Verification items for the finished model (mm, model axes). A direction names the side the tool comes from. Give positions to 0.01 mm unless a question says otherwise; leave off trailing zeros. Order: outer loops, then holes, each group sorted by start corner. A loop starts at its lowest first (then second) coordinate and runs counter-clockwise, first axis right, second up. Notation, with made-up numbers: (58, -28.75) - (96, -28.75) arc R14 ccw to (96, -4.75) - close; hole circle Ø6 at (11, 22.5). An arc over 180 degrees is marked (long way). Answer as a JSON object with one key per item and string values.
```python
from build123d import *

# Parameters (mm, degrees)
SALIENTE_EXTRUIR1_DEPTH = 60
CHAFL_N1_SIZE           = 1.5
CROQUIS3_R              = 2.25
CORTAR_EXTRUIR2_DEPTH   = 4.5


with BuildPart() as part:
    # Croquis1 → Saliente-Extruir1 (new body, symmetric)
    with BuildSketch(Plane(origin=(0, 0, 0), x_dir=(0, 0, -1), z_dir=(1, 0, 0))):
        Polygon((0, -23.75), (0, 23.75), (-21, 23.75), (-21, 20.25), (-3.5, 20.25), (-3.5, -20.25), (-21, -20.25), (-21, -23.75), align=None)
    extrude(amount=SALIENTE_EXTRUIR1_DEPTH, both=True)

    # Chaflán1
    chafl_n1_edges = [part.edges().sort_by_distance(p)[0] for p in [
        (0, 23.75, 0),
        (0, -23.75, 0),
    ]]
    chamfer(chafl_n1_edges, length=CHAFL_N1_SIZE)

    # Croquis3 → Cortar-Extruir2 (cut, through all)
    with BuildSketch(Plane.XY.offset(3.5)):
        with Locations((-40, 0.25)):
            Circle(CROQUIS3_R)
        with Locations((40, 0.25)):
            Circle(CROQUIS3_R)
    extrude(amount=-CORTAR_EXTRUIR2_DEPTH, mode=Mode.SUBTRACT)


solid = part.part
```
(1) Section check A-A (z = 10.5). Record the cut outline in (x, y), then the cut area to 3 significant figures.
Computed values:
{"outline": "(-60, -23.75) - (60, -23.75) - (60, -20.25) - (-60, -20.25) - close; (-60, 20.25) - (60, 20.25) - (60, 23.75) - (-60, 23.75) - close", "area": "840 mm²"}
(2) Section check D-D (x = 34). Record the cut outline in (y, z).
Computed values:
{"outline": "(-23.75, 1.5) - (-22.25, 0) - (22.25, 0) - (23.75, 1.5) - (23.75, 21) - (20.25, 21) - (20.25, 3.5) - (-20.25, 3.5) - (-20.25, 21) - (-23.75, 21) - close"}
(3) Access from +Z, -Z, +X, -X, +Y, -Y to the whole of each face (thin tool, end or side, straight path). Record for faces 5 (the flat face through (1, 23.75, 11)), 6 (the flat face through (1, 20.25, 12)).
Computed values:
{"face 5": "+Z, -Z, +X, -X, +Y", "face 6": "+Z, +X, -X"}
(4) Release check for a two-part mould opening along Y. For faces 1 (the cylindrical face through (-42.248, 0.349, 1.774)), 2 (the flat face through (60, -2, 3)), 3 (the flat face through (1, -23.75, 11)), 4 (the flat face through (1, 0, 3.5)) record: pulls with the +Y half, pulls with the -Y half, needs draft (parallel to the pull), parting line crosses it, or undercut.
Computed values:
{"face 1": "undercut", "face 2": "needs draft", "face 3": "pulls with the -Y half", "face 4": "undercut"}
(5) Section check B-B (x = -40). Record the cut outline in (y, z).
Computed values:
{"outline": "(-23.75, 1.5) - (-22.25, 0) - (-2, 0) - (-2, 3.5) - (-20.25, 3.5) - (-20.25, 21) - (-23.75, 21) - close; (2.5, 0) - (22.25, 0) - (23.75, 1.5) - (23.75, 21) - (20.25, 21) - (20.25, 3.5) - (2.5, 3.5) - close"}
(6) Gauge pin test, flat ends, axial feed: pin 1 Ø4 at (x, y) = (40, 0.25) entering from -Z; pin 2 Ø6 at (y, z) = (17.5, 7.5) entering from +X; pin 3 Ø6 at (x, y) = (-40, 0.25) entering from +Z. Record the tip position at first contact, or that the pin passes through.
Computed values:
{"pin 1": "passes through", "pin 2": "stops at x = 60", "pin 3": "stops at z = 3.5"}
(7) Material ranges on line 1 along Y through (x, z) = (24.5, 9.75); line 2 along Y through (x, z) = (-40, 1.6); line 3 along Z through (x, y) = (53, 14.5), recorded low to high. Write a range as [from, to].
Computed values:
{"line 1": "y = [-23.75, -20.25], [20.25, 23.75]", "line 2": "y = [-23.75, -2], [2.5, 23.75]", "line 3": "z = [0, 3.5]"}
(8) Section check C-C (y = 0.25). Record the cut outline in (x, z), then the cut area to 4 significant figures.
Computed values:
{"outline": "(-60, 0) - (-42.25, 0) - (-42.25, 3.5) - (-60, 3.5) - close; (-37.75, 0) - (37.75, 0) - (37.75, 3.5) - (-37.75, 3.5) - close; (42.25, 0) - (60, 0) - (60, 3.5) - (42.25, 3.5) - close", "area": "388.5 mm²"}
